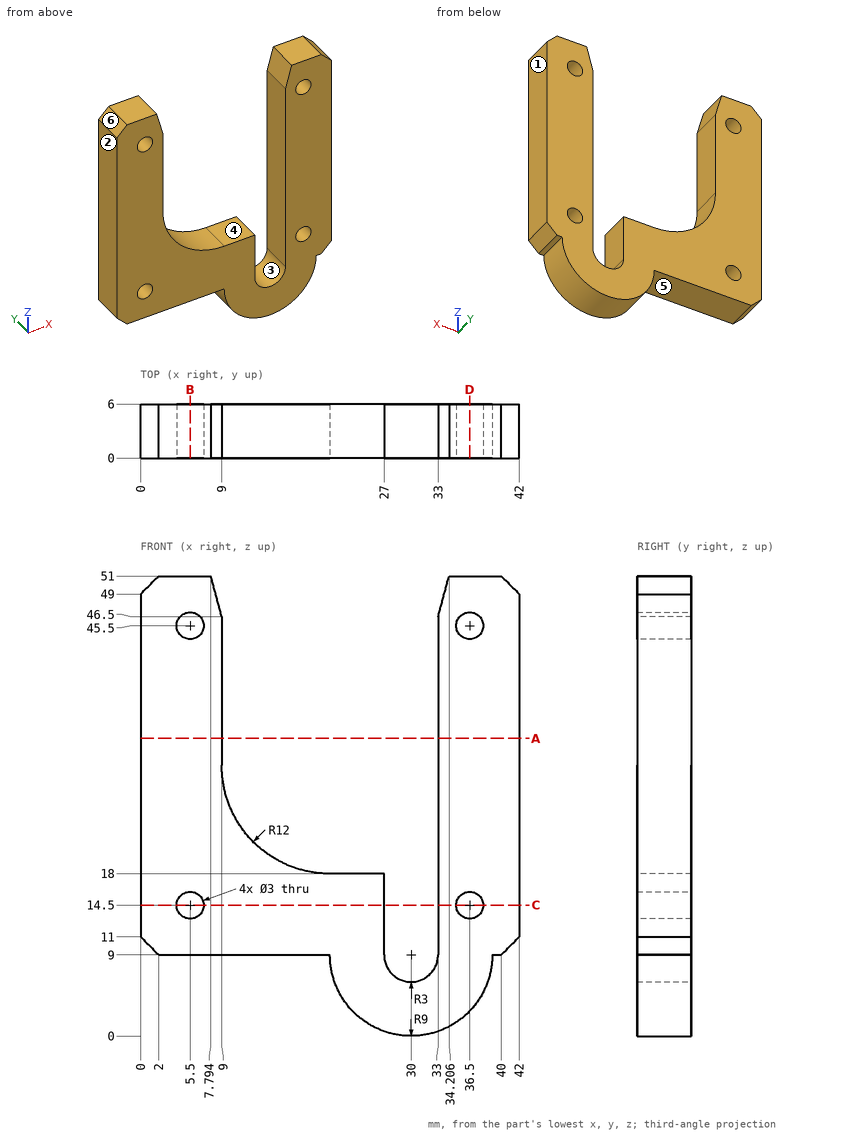
Here's the drawing with two shaded views (mm, measured from the low corner). I have some questions. A direction names the side the tool comes from. Round coordinates to 2 decimals unless told otherwise and drop trailing zeros. Loops run counter-clockwise (first coordinate to the right, second up) from the corner with the lowest first, then second, coordinate; pieces in that order, holes last. Notation, with made-up numbers: M 60.25,-5 L 79.25,-5 A21 cw 79.25,32 Z; hole C -26.5,-28.75 d11. An arc over 180 degrees is marked long. Answer as a JSON object with one key per item and string values. Group by question number.
Q1. On a 3-axis mill with a long thin cutter (end or side, diameter ignored), from which of +Z, -Z, +X, -X, +Y, -Y can I reach the whole of each face in a straight line? I mean the marked faces 4, 5 and 6. Say none if no direction works.
Q2. Imagine slicing it at C-C, the plane z = 14.5. Please give me the cut outline in (x, y).
Q3. Please list where these lines run through material, in increasing order: L1, parallel to X at y = 1.8, z = 14.5; L2, parallel to X at y = 3.1, z = 45.5; L3, parallel to X at y = 4.3, z = 29.5.
Q4. Imagine slicing it at D-D, the plane x = 36.5. Please give me the cut outline in (y, z) (1 decimal), then the cut area to 3 significant figures.
Q5. Imagine slicing it at B-B, the plane x = 5.5. Please give me the cut outline in (y, z).
Q6. Imagine slicing it at A-A, the plane z = 33. Please give me the cut outline in (x, y), then the cut area to 3 significant figures.
Q7. Will these pins go through, and if not, where does the flat tip stop? pin 1 (2.5 mm diameter, centred on x = 5.5, z = 14.5, fed in from +Y); pin 2 (2 mm diameter, centred on x = 36, y = 1, fed in from -Z); pin 3 (0.5 mm diameter, centred on x = 39.5, y = 3.5, fed in from -Z).
Q8. We'd pull the mould along X, two halves only. Please class the marked faces 1, 2 and 3: +X half, -X half, draft (parallel to the pull), parting line (faces both ways), or undercut.
Findings:
{
 "1": {"face 4": "+Z, +Y, -Y", "face 5": "-Z, -X, +Y, -Y", "face 6": "+Z, -X, +Y, -Y"},
 "2": {"outline": "M 0,0 L 4,0 L 4,6 L 0,6 Z; M 7,0 L 27,0 L 27,6 L 7,6 Z; M 33,0 L 35,0 L 35,6 L 33,6 Z; M 38,0 L 42,0 L 42,6 L 38,6 Z"},
 "3": {"L1": "x = 0 to 4, 7 to 27, 33 to 35, 38 to 42", "L2": "x = 0 to 4, 7 to 9, 33 to 35, 38 to 42", "L3": "x = 0 to 9.01, 33 to 42"},
 "4": {"outline": "M 0,2.8 L 6,2.8 L 6,13 L 0,13 Z; M 0,16 L 6,16 L 6,44 L 0,44 Z; M 0,47 L 6,47 L 6,51 L 0,51 Z", "area": "253 mm2"},
 "5": {"outline": "M 0,9 L 6,9 L 6,13 L 0,13 Z; M 0,16 L 6,16 L 6,44 L 0,44 Z; M 0,47 L 6,47 L 6,51 L 0,51 Z"},
 "6": {"outline": "M 0,0 L 9,0 L 9,6 L 0,6 Z; M 33,0 L 42,0 L 42,6 L 33,6 Z", "area": "108 mm2"},
 "7": {"pin 1": "passes through", "pin 2": "stops at z = 1.52", "pin 3": "stops at z = 9"},
 "8": {"face 1": "+X half", "face 2": "-X half", "face 3": "undercut"}
}
